Part model, mm, in its own coordinate system. A direction names the side the tool comes from. Round coordinates to 2 decimals unless told otherwise and drop trailing zeros. Loops run counter-clockwise (first coordinate to the right, second up) from the corner with the lowest first, then second, coordinate; pieces in that order, holes last. Notation, with made-up numbers: M 28,-38.75 L 57,-38.75 A20 ccw 57,-19.75 Z; hole C 81,-39.75 d7. An arc over 180 degrees is marked long. Put each result on its own line as item: value. Start each with the question number.
1) Slice it at C-C on y = 8. Give the cut face in (x, z), then the cut area to 3 significant figures.
2) Probe line 1 along Y through (x, z) = (23, 5.75); line 2 along Y through (x, z) = (10, 3); line 3 along X through (y, z) = (10, 7.5). List the from-to ranges inside material, lowest first.
3) Slice it at D-D on z = 5.5. Give the cut face in (x, y), then the cut area to 3 significant figures.
4) Which spindle directions (+Z, -Z, +X, -X, +Y, -Y) get a long thin tool onto all of the face, cutting with end or side? Do faces 4 (the flat face through (28.817, 12, 5)), 5 (the flat face through (23, 8, 4)). Say none if no direction does.
5) Pull direction Y, two halves, no side cores. Call faces 1 (the cylindrical face through (22.42, 5.56, 7.04)), 2 (the flat face through (14, 12, 10)), 3 (the flat face through (14, 0, 5)): +Y half, -Y half, draft (parallel to the pull), parting line (faces both ways), or undercut.
6) Slice it at B-B on z = 1. Give the cut face in (x, y).
7) Slice it at A-A on x = 10. Give the cut face in (y, z).
```python
from build123d import *

# Parameters (mm, degrees)
SKETCH_W        = 28.817356
SKETCH_H        = 24.401199
PAD_DEPTH       = 10
SKETCH001_R     = 4
POCKET_DEPTH    = 10.001
SKETCH002_R     = 2.5
POCKET001_DEPTH = 6


with BuildPart() as part:
    # Sketch → Pad (new body)
    with BuildSketch(Plane.XY):
        with Locations((14.408678, 12.200599)):
            Rectangle(SKETCH_W, SKETCH_H)
    extrude(amount=PAD_DEPTH)

    # Sketch001 → Pocket (cut, through all)
    with BuildSketch(Plane.XY):
        with Locations((10, 10)):
            Circle(SKETCH001_R)
    extrude(amount=POCKET_DEPTH, mode=Mode.SUBTRACT)

    # Sketch002 (on Face5 of Pocket) → Pocket001 (cut)
    with BuildSketch(Plane.XY.offset(10)):
        with Locations((22.960093, 8)):
            Circle(SKETCH002_R)
        with Locations((22.960093, 20)):
            Circle(SKETCH002_R)
    extrude(amount=-POCKET001_DEPTH, mode=Mode.SUBTRACT)


solid = part.part
```
Recorded:
1. outline: M 0,0 L 6.54,0 L 6.54,10 L 0,10 Z; M 13.46,0 L 28.82,0 L 28.82,10 L 25.46,10 L 25.46,4 L 20.46,4 L 20.46,10 L 13.46,10 Z
1. area: 189 mm2
2. line 1: y = 0 to 5.5, 10.5 to 17.5, 22.5 to 24.4
2. line 2: y = 0 to 6, 14 to 24.4
2. line 3: x = 0 to 6, 14 to 21.46, 24.46 to 28.82
3. outline: M 0,0 L 28.82,0 L 28.82,24.4 L 0,24.4 Z; hole C 10,10 d8; hole C 22.96,8 d5; hole C 22.96,20 d5
3. area: 614 mm2
4. face 4: +Z, -Z, +X, +Y, -Y
4. face 5: +Z
5. face 1: undercut
5. face 2: draft
5. face 3: -Y half
6. outline: M 0,0 L 28.82,0 L 28.82,24.4 L 0,24.4 Z; hole C 10,10 d8
7. outline: M 0,0 L 6,0 L 6,10 L 0,10 Z; M 14,0 L 24.4,0 L 24.4,10 L 14,10 Z
